Part model, mm, in its own coordinate system. A direction names the side the tool comes from. Give positions to 0.01 mm unless a question says otherwise; leave off trailing zeros. Order: outer loops, then holes, each group sorted by start corner. A loop starts at its lowest first (then second) coordinate and runs counter-clockwise, first axis right, second up.
1. Which spindle directions (+Z, -Z, +X, -X, +Y, -Y) get a long thin tool onto all of the face, cutting with end or side? Do faces 4 (the flat face through (-26, 6, 21.875)), 5 (the flat face through (-28, 11.25, -4)). Say none if no direction does.
2. Probe line 1 (X direction, y = 10, z = 26) (3 decimals); line 2 (Z direction, x = 12.5, y = 8.75) (3 decimals); line 3 (X direction, y = 6.25, z = 24) (3 decimals). List the from-to ranges inside material, lowest first.
3. Slice it at A-A on x = -9.5. List the corners of the cut face in (y, z) (3 decimals), and give its area (3 significant figures).
4. Slice it at B-B on z = -18.5. List the corners of the cut face in (x, y) (3 decimals), and give its area (3 significant figures).
5. Slice it at C-C on y = 5. List the corners of the cut face in (x, z) (3 decimals).
6. Mould opens along Z. For faces 1 (the flat face through (-31.375, 6, 1)), 2 (the flat face through (-24, 4, 24)), 3 (the flat face through (0, 6, 46.125)) say: +Z half, -Z half, draft (parallel to the pull), parting line (faces both ways), or undercut.
7. Drop flat-ended pins along their axis: pin 1 Ø6 at (x, z) = (1.5, 27) entering from +Y; pin 2 Ø4 at (x, z) = (24.5, 39) entering from +Y. Give the stop position or say it passes through.
from build123d import *

# Parameters (mm, degrees)
SKETCH1_W           = 62.75
SKETCH1_H           = 92.25
BOSS_EXTRUDE1_DEPTH = 4
SKETCH2_W           = 62.75
SKETCH2_H           = 92.25
SKETCH2_W_2         = 54.75
SKETCH2_H_2         = 84.25
BOSS_EXTRUDE2_DEPTH = 7.25
SKETCH3_R           = 0.85
BOSS_EXTRUDE3_DEPTH = 5


with BuildPart() as part:
    # Sketch1 → Boss-Extrude1 (new body)
    with BuildSketch(Plane(origin=(0, 0, 0), x_dir=(1, 0, 0), z_dir=(0, 1, 0))):
        Rectangle(SKETCH1_W, SKETCH1_H)
    extrude(amount=BOSS_EXTRUDE1_DEPTH)

    # Sketch2 → Boss-Extrude2 (add)
    with BuildSketch(Plane(origin=(0, 4, 0), x_dir=(1, 0, 0), z_dir=(0, 1, 0))):
        Rectangle(SKETCH2_W, SKETCH2_H)
        Rectangle(SKETCH2_W_2, SKETCH2_H_2, mode=Mode.SUBTRACT)
    extrude(amount=BOSS_EXTRUDE2_DEPTH)

    # Sketch3 → Boss-Extrude3 (add)
    with BuildSketch(Plane(origin=(0, 4, 0), x_dir=(1, 0, 0), z_dir=(0, 1, 0))):
        with BuildLine():
            Line((-21.375, 39.175), (-21.375, 42.125))
            Line((-21.375, 42.125), (-27.375, 42.125))
            Line((-27.375, 42.125), (-27.375, 36.675))
            Line((-27.375, 36.675), (-23.875, 36.675))
            ThreePointArc((-23.875, 36.675), (-22.107233047, 37.407233047), (-21.375, 39.175))
        make_face()
        with Locations((-23.875, 39.175)):
            Circle(SKETCH3_R, mode=Mode.SUBTRACT)
        with BuildLine():
            Line((22.125, 39.125), (22.125, 42.125))
            Line((22.125, 42.125), (27.375, 42.125))
            Line((27.375, 42.125), (27.375, 36.625))
            Line((27.375, 36.625), (24.625, 36.625))
            ThreePointArc((24.625, 36.625), (22.857233047, 37.357233047), (22.125, 39.125))
        make_face()
        with Locations((24.625, 39.125)):
            Circle(SKETCH3_R, mode=Mode.SUBTRACT)
        with BuildLine():
            Line((22.375, -39.575), (22.375, -42.125))
            Line((22.375, -42.125), (27.375, -42.125))
            Line((27.375, -42.125), (27.375, -37.075))
            Line((27.375, -37.075), (24.875, -37.075))
            ThreePointArc((24.875, -37.075), (23.107233047, -37.807233047), (22.375, -39.575))
        make_face()
        with Locations((24.875, -39.575)):
            Circle(SKETCH3_R, mode=Mode.SUBTRACT)
        with BuildLine():
            Line((-23.875, -26.875), (-27.375, -26.875))
            Line((-27.375, -26.875), (-27.375, -21.875))
            Line((-27.375, -21.875), (-23.875, -21.875))
            ThreePointArc((-23.875, -21.875), (-21.375, -24.375), (-23.875, -26.875))
        make_face()
        with Locations((-23.875, -24.375)):
            Circle(SKETCH3_R, mode=Mode.SUBTRACT)
    extrude(amount=BOSS_EXTRUDE3_DEPTH)


solid = part.part
Data:
1. face 4: +Y
1. face 5: +Z, -Z, +X, -X, +Y
2. line 1: x = -31.375 to -27.375, 27.375 to 31.375
2. line 2: z = -46.125 to -42.125, 42.125 to 46.125
2. line 3: x = -31.375 to -24.638, -23.112 to -21.403, 27.375 to 31.375
3. outline: (0, -46.125) - (11.25, -46.125) - (11.25, -42.125) - (4, -42.125) - (4, 42.125) - (11.25, 42.125) - (11.25, 46.125) - (0, 46.125) - close
3. area: 427 mm2
4. outline: (-31.375, 0) - (31.375, 0) - (31.375, 11.25) - (27.375, 11.25) - (27.375, 4) - (-27.375, 4) - (-27.375, 11.25) - (-31.375, 11.25) - close
4. area: 309 mm2
5. outline: (-31.375, -46.125) - (31.375, -46.125) - (31.375, 46.125) - (-31.375, 46.125) - close; hole (-27.375, -36.675) - (-23.875, -36.675) arc R2.5 cw to (-21.375, -39.175) - (-21.375, -42.125) - (22.125, -42.125) - (22.125, -39.125) arc R2.5 cw to (24.625, -36.625) - (27.375, -36.625) - (27.375, 37.075) - (24.875, 37.075) arc R2.5 cw to (22.375, 39.575) - (22.375, 42.125) - (-27.375, 42.125) - (-27.375, 26.875) - (-23.875, 26.875) arc R2.5 cw to (-23.875, 21.875) - (-27.375, 21.875) - close; hole circle Ø1.7 at (-23.875, -39.175); hole circle Ø1.7 at (-23.875, 24.375); hole circle Ø1.7 at (24.625, -39.125); hole circle Ø1.7 at (24.875, 39.575)
6. face 1: draft
6. face 2: undercut
6. face 3: +Z half
7. pin 1: stops at y = 4
7. pin 2: stops at y = 9
